Build history of the part. All positions in model axes, mm. A direction names the side the tool comes from. Give positions to 0.01 mm unless a question says otherwise; leave off trailing zeros. Order: outer loops, then holes, each group sorted by start corner. A loop starts at its lowest first (then second) coordinate and runs counter-clockwise, first axis right, second up. Notation, with made-up numbers: (61, -3) -> (83, -3) arc R25 ccw to (83, 24) -> close; hole circle Ø11 at (63.5, 66.5). An arc over 180 degrees is marked (long way). One line per item, written item: value. Start each with the question number.
(1) Saw through at B-B on z = 3.15. Give the cut face in (x, y), plus the area to 3 significant figures.
(2) Which spindle directions (+Z, -Z, +X, -X, +Y, -Y) get a long thin tool onto all of the face, cutting with end or side? Do faces 1 (the flat face through (0, -15, 3.5)), 2 (the cylindrical face through (-1.11, 16.01, 2.74)). Say none if no direction does.
(3) Pin check, flat tips, straight feed: pin 1 (1.5 mm diameter, centred on x = -2, z = 1, fed in from +Y); pin 2 (1.5 mm diameter, centred on x = 1.5, z = 0.5, fed in from -Y). Stop position of each tip, or through.
(4) Two-plate mould, pull along Y, no slides. Class faces 3 (the cylindrical face through (-0.325, -16.464, 2.74)), 4 (the cylindrical face through (0, -2, 1)), 5 (the cylindrical face through (2.797, 17.359, 1.014)), 6 (the cylindrical face through (2.797, -17.359, 1.014)): +Y half, -Y half, draft (parallel to the pull), parting line (faces both ways), or undercut.
(5) Saw through at A-A on y = 0. Give the cut face in (x, z).
(6) Saw through at D-D on y = -15.5. Give the cut face in (x, z), plus the area to 3 significant figures.
(7) Saw through at C-C on x = -0.5. Give the cut face in (y, z), plus the area to 3 significant figures.
(8) Probe line 1 (Y direction, x = 0, z = 1.15); line 2 (Z direction, x = -3, y = 16); line 3 (Y direction, x = 1.75, z = 1.95). List the from-to ranges inside material, lowest first.
```python
from build123d import *

# Parameters (mm, degrees)
F0_W     = 8
F0_H     = 37
F0_R     = 2
F1_DEPTH = 2
F2_R     = 1.5
F3_DEPTH = 1.5
F4_R     = 3.99999


# Not quite as in the source:
# - a fillet or chamfer is up to 0.001 mm smaller than in the source, because OpenCascade refuses the exact size


with BuildPart() as f1:
    # F0 (on Top) → F1 (new body)
    with BuildSketch(Plane.XY):
        Rectangle(F0_W, F0_H)
        Circle(F0_R, mode=Mode.SUBTRACT)
    extrude(amount=F1_DEPTH)

    # F2 (on face) → F3 (join)
    with BuildSketch(Plane.XY.offset(2)):
        with Locations((0, 15)):
            Circle(F2_R)
        with Locations((0, -15)):
            Circle(F2_R)
    extrude(amount=F3_DEPTH)

    # F4 (radius 4 in the source; OpenCascade refuses exactly that, so slightly less here)
    f4_edges = [f1.edges().sort_by_distance(p)[0] for p in [
        (-4, 18.5, 1),
        (4, 18.5, 1),
        (4, -18.5, 1),
        (-4, -18.5, 1),
    ]]
    fillet(f4_edges, radius=F4_R)


solid = f1.part
```
Results below:
1. outline: circle Ø3 at (0, -15); circle Ø3 at (0, 15)
1. area: 14.1 mm²
2. face 1: +Z, +X, -X, +Y, -Y
2. face 2: +Z
3. pin 1: stops at y = 18.3
3. pin 2: stops at y = -18.43
4. face 3: undercut
4. face 4: undercut
4. face 5: +Y half
4. face 6: -Y half
5. outline: (-4, 0) -> (-2, 0) -> (-2, 2) -> (-4, 2) -> close; (2, 0) -> (4, 0) -> (4, 2) -> (2, 2) -> close
6. outline: (-3.87, 0) -> (3.87, 0) -> (3.87, 2) -> (1.41, 2) -> (1.41, 3.5) -> (-1.41, 3.5) -> (-1.41, 2) -> (-3.87, 2) -> close
6. area: 19.7 mm²
7. outline: (-18.47, 0) -> (-1.94, 0) -> (-1.94, 2) -> (-13.59, 2) -> (-13.59, 3.5) -> (-16.41, 3.5) -> (-16.41, 2) -> (-18.47, 2) -> close; (1.94, 0) -> (18.47, 0) -> (18.47, 2) -> (16.41, 2) -> (16.41, 3.5) -> (13.59, 3.5) -> (13.59, 2) -> (1.94, 2) -> close
7. area: 74.6 mm²
8. line 1: y = -18.5 to -2, 2 to 18.5
8. line 2: z = 0 to 2
8. line 3: y = -18.1 to -0.97, 0.97 to 18.1
